For this review, use the dimensioned drawing (mm, ordinates from the lowest corner) and the shaded views. A direction names the side the tool comes from. Round coordinates to 2 decimals unless told otherwise and drop trailing zeros. Order: outer loops, then holes, each group sorted by start corner. A loop starts at its lowest first (then second) coordinate and runs counter-clockwise, first axis right, second up. Notation, with made-up numbers: M -17.75,57.5 L 20.25,57.5 A28 ccw 20.25,77.5 Z; hole C 33.5,86 d7. An arc over 180 degrees is marked long. Use a Markdown table: item, result. Add a question column.
1. Consider section B-B on z = 4.75. State the section outline as (x, y) points.
2. Consider section D-D on x = 60. State the section outline as (y, z) points.
3. To check wall thickness, follow probe 1 along Y at (x, z) = (6, 6.25); probe 2 along X at (y, z) = (90, 4.25); probe 3 along Y at (x, z) = (60, 4.25). State the ranges of each line that lie inside material, in increasing order.
4. Insertion check: P1, Ø4.5, axis at x = 6, y = 10, coming from the -Z side; P2, Ø3, axis at x = 51.5, z = 5, coming from the -Y side; P3, Ø5, axis at x = 51, z = 7, coming from the +Y side; P4, Ø4, axis at x = 72.5, z = 5, coming from the -Y side. Each pin has a flat end and moves straight along its axis. Give the tip position at first contact, or say it passes through.
5. Consider section C-C on y = 87. State the section outline as (x, z) points.
6. Consider section A-A on y = 10. State the section outline as (x, z) points, then the cut area to 3 significant figures.
7. For the marked faces 1, 2 and 3, list the 3-axis set-ups (+Z, -Z, +X, -X, +Y, -Y) from which the entire face can be reached by the end or side of a thin tool; tool diameter is ignored.
8. The part is to be moulded in two halves that separate along X. For the marked faces 4, 5 and 6, say which applies: +X half, -X half, draft (parallel to the pull), parting line (faces both ways), or undercut.
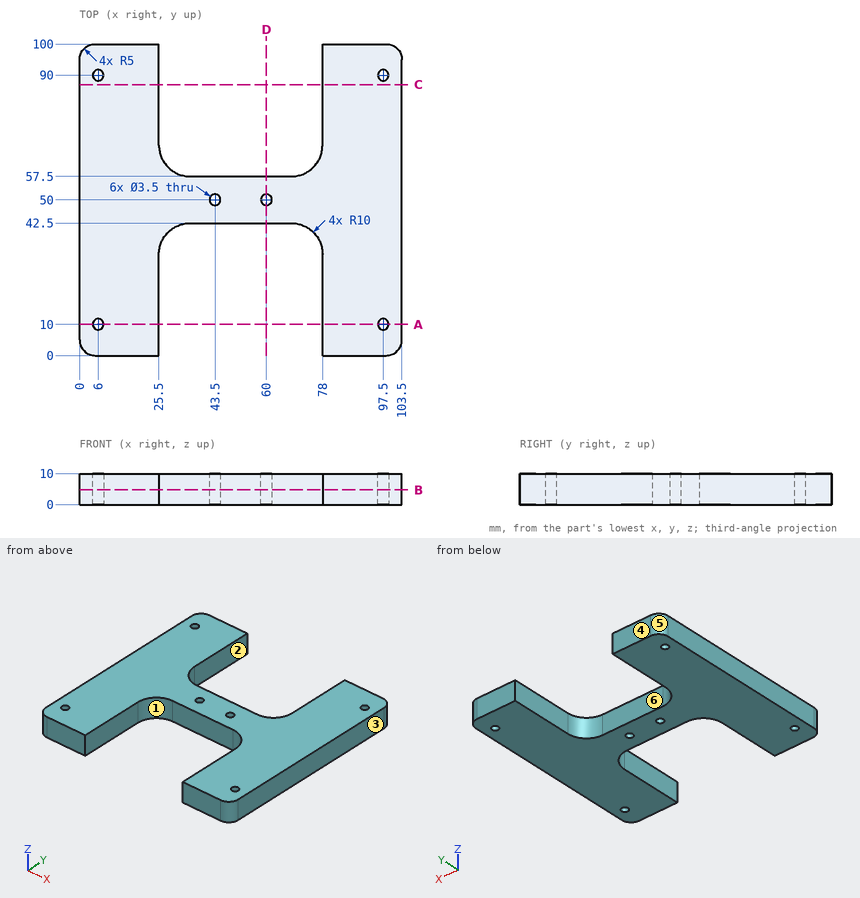
Answer block:
| question | item | result |
|---|---|---|
| 1 | outline | M 0,5 A5 ccw 5,0 L 25.5,0 L 25.5,32.5 A10 cw 35.5,42.5 L 68,42.5 A10 cw 78,32.5 L 78,0 L 98.5,0 A5 ccw 103.5,5 L 103.5,95 A5 ccw 98.5,100 L 78,100 L 78,67.5 A10 cw 68,57.5 L 35.5,57.5 A10 cw 25.5,67.5 L 25.5,100 L 5,100 A5 ccw 0,95 Z; hole C 6,10 d3.5; hole C 6,90 d3.5; hole C 43.5,50 d3.5; hole C 60,50 d3.5; hole C 97.5,10 d3.5; hole C 97.5,90 d3.5 |
| 2 | outline | M 42.5,0 L 48.25,0 L 48.25,10 L 42.5,10 Z; M 51.75,0 L 57.5,0 L 57.5,10 L 51.75,10 Z |
| 3 | probe 1 | 0 to 8.25, 11.75 to 88.25, 91.75 to 100 |
| 3 | probe 2 | 0 to 4.25, 7.75 to 25.5, 78 to 95.75, 99.25 to 103.5 |
| 3 | probe 3 | 42.5 to 48.25, 51.75 to 57.5 |
| 4 | P1 | z = 0 |
| 4 | P2 | y = 42.5 |
| 4 | P3 | y = 57.5 |
| 4 | P4 | y = 40.1 |
| 5 | outline | M 0,0 L 25.5,0 L 25.5,10 L 0,10 Z; M 78,0 L 103.5,0 L 103.5,10 L 78,10 Z |
| 6 | outline | M 0,0 L 4.25,0 L 4.25,10 L 0,10 Z; M 7.75,0 L 25.5,0 L 25.5,10 L 7.75,10 Z; M 78,0 L 95.75,0 L 95.75,10 L 78,10 Z; M 99.25,0 L 103.5,0 L 103.5,10 L 99.25,10 Z |
| 6 | area | 440 mm^2 |
| 7 | face 1 | +Z, -Z, -Y |
| 7 | face 2 | +Z, -Z, +Y |
| 7 | face 3 | +Z, -Z, +X, +Y, -Y |
| 8 | face 4 | draft |
| 8 | face 5 | -X half |
| 8 | face 6 | undercut |
